Source: CAD feature listing. Evaluate the final solid. Frame: model axes, mm. A direction names the side the tool comes from. Coordinates: 2 decimals unless noted, no trailing zeros. Loops run counter-clockwise (first coordinate to the right, second up) from the corner with the lowest first, then second, coordinate; pieces in that order, holes last.
Item 1: Section query D-D, the plane y = 3.5. Return the cut outline in (x, z), then the cut area to 3 significant figures.
Item 2: Reachability of faces 4 (the cylindrical face through (1.22, 2.96, 0.27)), 5 (the flat face through (0, 0, 0)), 6 (the flat face through (1, 7, -0.375)) from +Z, -Z, +X, -X, +Y, -Y: full face, straight path, thin tool, end or side. Return the list, or none.
Item 3: Section query C-C, the plane z = 0. Return the cut outline in (x, y).
Item 4: Pin query (flat end, axial travel): pin 1 Ø0.7 at (x, y) = (-1, 6.5) entering from +Z; pin 2 Ø0.9 at (x, y) = (1, 7) entering from -Z; pin 3 Ø0.7 at (y, z) = (7, -0.5) entering from +X. Return the tip coordinate at first contact, or that it passes through.
Item 5: Section query A-A, the plane y = 6.75. Return the cut outline in (x, z) (3 decimals), then the cut area to 3 significant figures.
Item 6: Line query: probe 1 along Y at (x, z) = (0.2, -1.1); probe 2 along Y at (x, z) = (-1.2, -0.85); probe 3 along Z at (x, y) = (1, 6.5) (3 decimals). Output: solid intervals per line, ascending.
Item 7: Section query B-B, the plane x = 0. Return the cut outline in (y, z).
Item 8: Pull-direction query (Z, two-part tool) for faces 1 (the flat face through (-1, 6, -1)), 2 (the flat face through (0, 6.45, 0)), 3 (the cylindrical face through (2, 7, 0)); classes: +Z half, -Z half, draft (parallel to the pull), parting line (faces both ways), or undercut.
```python
from build123d import *

# Parameters (mm, degrees)
CUT_EXTRUDE1_DEPTH = 0.85


with BuildPart() as part:
    # Sketch1 → Revolve1 (revolve)
    with BuildSketch(Plane(origin=(0, 0, 0), x_dir=(0, 0, -1), z_dir=(1, 0, 0))):
        Polygon((0, 7.3), (2, 7.3), (2, 6), (1.25, 6), (1.25, 0), (0, 0), align=None)
    revolve(axis=Axis((0, 0, 0), (0, 1, 0)))

    # Sketch4 → Cut-Extrude1 (cut)
    with BuildSketch(Plane(origin=(0, 7.3, 0), x_dir=(1, 0, 0), z_dir=(0, 1, 0))):
        Polygon((0.375, -0.375), (0.375, -1.3), (-0.375, -1.3), (-0.375, -0.375), (-1.3, -0.375), (-1.3, 0.375), (-0.375, 0.375), (-0.375, 1.3), (0.375, 1.3), (0.375, 0.375), (1.3, 0.375), (1.3, -0.375), align=None)
    extrude(amount=-CUT_EXTRUDE1_DEPTH, mode=Mode.SUBTRACT)


solid = part.part
```
Verdict:
1. outline: circle Ø2.5 at (0, 0)
1. area: 4.91 mm2
2. face 4: -Y
2. face 5: +Z, -Z, +X, -X, -Y
2. face 6: +Y
3. outline: (-2, 6) - (-1.25, 6) - (-1.25, 0) - (1.25, 0) - (1.25, 6) - (2, 6) - (2, 7.3) - (1.3, 7.3) - (1.3, 6.45) - (-1.3, 6.45) - (-1.3, 7.3) - (-2, 7.3) - close
4. pin 1: stops at z = 1.89
4. pin 2: stops at z = -1.92
4. pin 3: stops at x = 1.99
5. outline: circle Ø4 at (0, 0); hole (-1.3, -0.375) - (-0.375, -0.375) - (-0.375, -1.3) - (0.375, -1.3) - (0.375, -0.375) - (1.3, -0.375) - (1.3, 0.375) - (0.375, 0.375) - (0.375, 1.3) - (-0.375, 1.3) - (-0.375, 0.375) - (-1.3, 0.375) - close
5. area: 9.23 mm2
6. probe 1: y = 0 to 6.45
6. probe 2: y = 6 to 7.3
6. probe 3: z = -1.732 to -0.375, 0.375 to 1.732
7. outline: (0, -1.25) - (6, -1.25) - (6, -2) - (7.3, -2) - (7.3, -1.3) - (6.45, -1.3) - (6.45, 1.3) - (7.3, 1.3) - (7.3, 2) - (6, 2) - (6, 1.25) - (0, 1.25) - close
8. face 1: draft
8. face 2: undercut
8. face 3: parting line
